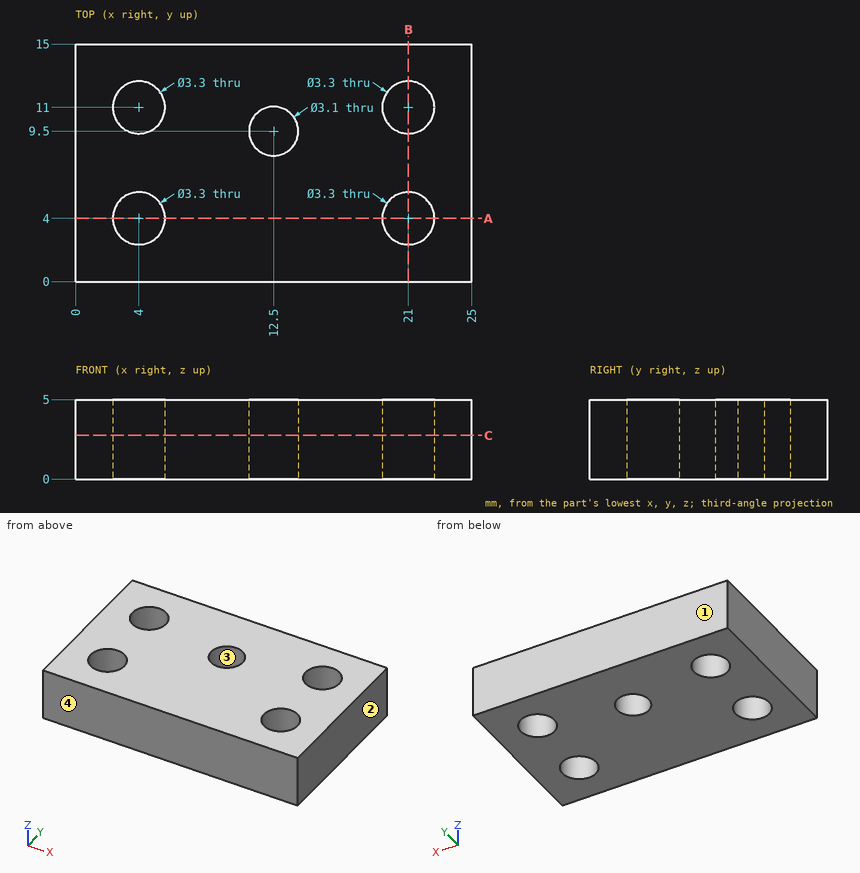
Geometry check sheet. Reference: drawing and pictorial views, mm from the part's lowest x, y, z. Coordinates: 2 decimals unless noted, no trailing zeros. Order: outer loops, then holes, each group sorted by start corner. A loop starts at its lowest first (then second) coordinate and runs counter-clockwise, first axis right, second up. Notation, with made-up numbers: (31, 26.5) -> (65, 26.5) arc R27 cw to (65, 54.5) -> close; hole circle Ø6 at (26.25, -23). An arc over 180 degrees is marked (long way). Use CSV: the item, a comma, the result in double quotes. Start each with the question number.
Q1. Section check A-A, the plane y = 4. Record the cut outline in (x, z).
Q2. Section check B-B, the plane x = 21. Record the cut outline in (y, z).
Q3. Section check C-C, the plane z = 2.75. Record the cut outline in (x, y), and give its area (3 significant figures).
Q4. Thickness scan on line 1 along Y through (x, z) = (21, 1.2); line 2 along X through (y, z) = (2.5, 1.5); line 3 along Y through (x, z) = (21.75, 2.8). Record the ranges inside material, lowest first.
Q5. Draft check along Y on the marked faces 1, 2, 3 and 4. Enter one of: +Y half, -Y half, draft (parallel to the pull), parting line (faces both ways), or undercut.
Returned:
1,outline,"(0, 0) -> (2.35, 0) -> (2.35, 5) -> (0, 5) -> close; (5.65, 0) -> (19.35, 0) -> (19.35, 5) -> (5.65, 5) -> close; (22.65, 0) -> (25, 0) -> (25, 5) -> (22.65, 5) -> close"
2,outline,"(0, 0) -> (2.35, 0) -> (2.35, 5) -> (0, 5) -> close; (5.65, 0) -> (9.35, 0) -> (9.35, 5) -> (5.65, 5) -> close; (12.65, 0) -> (15, 0) -> (15, 5) -> (12.65, 5) -> close"
3,outline,"(0, 0) -> (25, 0) -> (25, 15) -> (0, 15) -> close; hole circle Ø3.3 at (4, 4); hole circle Ø3.3 at (4, 11); hole circle Ø3.1 at (12.5, 9.5); hole circle Ø3.3 at (21, 4); hole circle Ø3.3 at (21, 11)"
3,area,"333 mm^2"
4,line 1,"y = 0 to 2.35, 5.65 to 9.35, 12.65 to 15"
4,line 2,"x = 0 to 3.31, 4.69 to 20.31, 21.69 to 25"
4,line 3,"y = 0 to 2.53, 5.47 to 9.53, 12.47 to 15"
5,face 1,"+Y half"
5,face 2,"draft"
5,face 3,"undercut"
5,face 4,"-Y half"
